Solid Edge part; units mm, degrees
sketch "Sketch1" plane through (0, 0, 0) normal (0, -1, 0) x (1, 0, 0)
  line L0 (12.5, 20) -> (12.5, 145)
  line L1 (12.5, 145) -> (15, 145)
  line L2 (15, 10) -> (15, 145)
  line L3 (7, 10) -> (15, 10)
  line L4 (7, 10) -> (7, 0)
  line L5 (1.6, 0) -> (7, 0)
  line L6 (1.6, 0) -> (1.6, 14)
  line L7 (1.6, 14) -> (0, 14)
  line L8 (0, 14) -> (0, 20)
  line L9 (0, 20) -> (12.5, 20)
revolve "RevolvedProtrusion1" add sketch "Sketch1" angle 360 about axis through (0, 0, 0) along (0, 0, 1)
sketch "Sketch2" plane through (0, 0, 145) normal (0, 0, 1) x (1, 0, 0)
  line L0 (0, 14.5) -> (0, 13)
  line L1 (0, 13) -> (1.299, 13.75)
  line L2 (1.299, 13.75) -> (0, 14.5)
extrude "ExtrudedProtrusion_1" add sketch "Sketch2" along normal blind 0.5
hole "Hole_1" at (7, 0, 5) direction (-1, 0, 0) diameter 2.459 end up to next thread major 3 thread length 2
properties material "Zinc"
Build history of the part. All positions in model axes, mm. A direction names the side the tool comes from. Round coordinates to 2 decimals unless told otherwise and drop trailing zeros. Write each loop counter-clockwise with the first axis right and the second up, starting at its lowest first coordinate (ties: lowest second). Pieces come first, ordered by that corner, then holes. Notation, with made-up numbers: (-15.75, 67.5) - (-1.75, 67.5) arc R21 cw to (-1.75, 81.5) - close; hole circle Ø11 at (71.25, 88). An arc over 180 degrees is marked (long way). One line per question, with ' | ' between items.
1. Drop flat-ended pins along their axis: pin 1 Ø15 at (x, y) = (5, -3) entering from -Z; pin 2 Ø3 at (x, y) = (8.5, -10) entering from +Z; pin 3 Ø4 at (x, y) = (0, 0) entering from +Z; pin 4 Ø2 at (x, z) = (-9.5, 44.5) entering from -Y. Give the stop position or say it passes through.
Results are:
pin 1: z = 0 | pin 2: z = 145 | pin 3: z = 20 | pin 4: y = -12.36
2. Band-saw the part on D-D, the plane y = -8.5. Write the cut outline in (x, z), and give its area (3 significant figures).
Results are:
outline: (-12.36, 10) - (12.36, 10) - (12.36, 145) - (9.17, 145) - (9.17, 20) - (-9.17, 20) - (-9.17, 145) - (-12.36, 145) - close | area: 1,050 mm^2
3. Band-saw the part on A-A, the plane y = 0. Write the cut outline in (x, z), and give its area (3 significant figures).
Results are:
outline: (-15, 10) - (-7, 10) - (-7, 0) - (-1.6, 0) - (-1.6, 14) - (1.6, 14) - (1.6, 6.23) - (7, 6.23) - (7, 10) - (15, 10) - (15, 145) - (12.5, 145) - (12.5, 20) - (-12.5, 20) - (-12.5, 145) - (-15, 145) - close; (1.6, 0) - (7, 0) - (7, 3.77) - (1.6, 3.77) - close | area: 1,010 mm^2
4. Band-saw the part on B-B, the plane z = 76.5. Write the cut outline in (x, y).
Results are:
outline: circle Ø30 at (0, 0); hole circle Ø25 at (0, 0)
5. Drill centre lines: line 1 along Y through (x, z) = (0, 49); line 2 along Z through (x, y) = (4.9, 0); line 3 along Y through (x, z) = (0, 10.25). Where is each one in solid material? Low to high. Write a range as from..to.
Results are:
line 1: -15..-12.5, 12.5..15 | line 2: 0..3.77, 6.23..20 | line 3: -15..-1.6, 1.6..15
6. Mould opens along Y. For faces 1 (the face through (3.1, -6.5, 10)), 2 (the face through (11.923, 3.755, 83.375)), 3 (the face through (6.466, 2.681, 4.93)) say: released by +Y, released by -Y, zero draft, split by the parting line, or undercut.
Results are:
face 1: zero draft | face 2: undercut | face 3: split by the parting line
7. Tool access for faces 4 (the face through (-14.985, 0.66, 78.445)), 5 (the face through (0, 0, 20)), 6 (the face through (0, 0, 14)), 7 (the face through (4.05, 1.22, 5.16)): list every direction of +Z, -Z, +X, -X, +Y, -Y with a clear straight run to the whole face (end or side of a thin tool).
Results are:
face 4: +Z, -Z | face 5: +Z | face 6: -Z | face 7: +X
8. Band-saw the part on C-C, the plane x = 4.25. Write the cut outline in (y, z).
Results are:
outline: (-14.39, 10) - (-5.56, 10) - (-5.56, 0) - (5.56, 0) - (5.56, 10) - (14.39, 10) - (14.39, 145) - (11.76, 145) - (11.76, 20) - (-11.76, 20) - (-11.76, 145) - (-14.39, 145) - close; hole circle Ø2.46 at (0, 5)
